Verification items for the finished model (mm, model axes). A direction names the side the tool comes from. Coordinates: 2 decimals unless noted, no trailing zeros. Write each loop counter-clockwise with the first axis right and the second up, starting at its lowest first coordinate (ties: lowest second). Pieces come first, ordered by that corner, then holes.
```python
from build123d import *

# Parameters (mm, degrees)
F1_DEPTH     = 10
F2_R         = 2
F3_DEPTH     = 115.001
F4_R         = 2
F4_R_2       = 1.25
F5_DEPTH     = 5
F6_R         = 2
F7_DEPTH     = 5
F9_DEPTH     = 10
F10_R        = 4.99999
F11_R        = 5
F12_DEPTH    = 10.001
F14_DEPTH    = 10
F15_T4_DEPTH = 78.4438958161
F15_T9_DEPTH = 78.4438958161
F16_R        = 4.99999


# Not quite as in the source:
# - a fillet or chamfer that OpenCascade refuses, or shapes differently, is made with other operations: its cross-section is extruded or revolved along the edge and cut away or added
# - a fillet or chamfer is up to 0.001 mm smaller than in the source, because OpenCascade refuses the exact size


with BuildPart() as f1:
    # F0 (on Front) → F1 (new body)
    with BuildSketch(Plane.XZ):
        Polygon((0, 115), (0, 0), (10, 0), (20, 0), (20, 5), (10, 5), (10, 110), (20, 110), (20, 115), (10, 115), align=None)
    extrude(amount=F1_DEPTH)

    # F2 (on face) → F3 (cut, through all)
    with BuildSketch(Plane.XY.offset(115)):
        with BuildLine():
            Line((0, -10), (5, -10))
            ThreePointArc((5, -10), (1.4644660941, -8.5355339059), (0, -5))
            Line((0, -5), (0, -10))
        make_face()
        with BuildLine():
            Line((0, 0), (0, -5))
            ThreePointArc((0, -5), (1.4644660941, -1.4644660941), (5, 0))
            Line((5, 0), (0, 0))
        make_face()
        with BuildLine():
            ThreePointArc((15.2, 0), (18.5941125497, -1.4058874503), (20, -4.8))
            Line((20, -4.8), (20, 0))
            Line((20, 0), (15.2, 0))
        make_face()
        with BuildLine():
            ThreePointArc((20, -5), (18.5355339059, -8.5355339059), (15, -10))
            Line((15, -10), (20, -10))
            Line((20, -10), (20, -5))
        make_face()
        with Locations((15, -5)):
            Circle(F2_R)
    extrude(amount=-F3_DEPTH, mode=Mode.SUBTRACT)

    # F4 (on face) → F5 (join)
    with BuildSketch(Plane.XY.offset(115)):
        with Locations((15, -5)):
            Circle(F4_R)
        with Locations((15, -5)):
            Circle(F4_R_2, mode=Mode.SUBTRACT)
    extrude(amount=-F5_DEPTH)

    # F6 (on face) → F7 (join)
    with BuildSketch(Plane(origin=(0, 0, 0), x_dir=(1, 0, 0), z_dir=(0, 0, -1))):
        with BuildLine():
            Line((-25, 0), (5, 0))
            ThreePointArc((5, 0), (0, 5), (5, 10))
            Line((5, 10), (-25, 10))
            ThreePointArc((-25, 10), (-28.5355339059, 8.5355339059), (-30, 5))
            ThreePointArc((-30, 5), (-28.5355339059, 1.4644660941), (-25, 0))
        make_face()
        with Locations((-25, 5)):
            Circle(F6_R, mode=Mode.SUBTRACT)
    extrude(amount=-F7_DEPTH)

    # F8 (on face) → F9 (join)
    with BuildSketch(Plane.XZ.offset(10)):
        Polygon((0, 115), (-20, 5), (5, 5), (5, 115), align=None)
    extrude(amount=-F9_DEPTH)

    # F10 (radius 5 in the source; OpenCascade refuses exactly that, so slightly less here)
    f10_edges = [f1.edges().sort_by_distance(p)[0] for p in [
        (-10, 0, 60),
        (-10, -10, 60),
    ]]
    fillet(f10_edges, radius=F10_R)

    # F11 (on face) → F12 (cut, through all)
    with BuildSketch(Plane.XZ.offset(10)):
        with Locations((0, 50.3422953188)):
            Circle(F11_R)
    extrude(amount=-F12_DEPTH, mode=Mode.SUBTRACT)

    # F13 (on face) → F14 (join)
    with BuildSketch(Plane(origin=(0, 0, 0), x_dir=(-1, 0, 0), z_dir=(0, 1, 0))):
        Polygon((-20, 110), (-10, 57.5), (-10, 110), (-15.2, 110), align=None)
    extrude(amount=-F14_DEPTH)

    # F15: fillet of radius 5 on 2 edges, made by hand


with BuildPart() as f15_tool2:
    # F15_s3 → F15_t4 (new body)
    with BuildSketch(Plane(origin=(23.2579385477, 0, 122.1041773757), x_dir=(0, 1, 0), z_dir=(-0.1871121079, 0, -0.9823385664))):
        with BuildLine():
            ThreePointArc((0, -5.9355605394), (-1.4644660941, -2.4000266335), (-5, -0.9355605394))
            Line((-5, -0.9355605394), (0, -0.9355605394))
            Line((0, -0.9355605394), (0, -5.9355605394))
        make_face()
    extrude(amount=F15_T4_DEPTH)

    split(bisect_by=Plane.YZ.offset(10), keep=Keep.TOP)


with BuildPart() as f1_1:
    add(f1.part)

    # F15_t1: cut F15_tool2
    add(f15_tool2.part, mode=Mode.SUBTRACT)


with BuildPart() as f15_tool7:
    # F15_s8 → F15_t9 (new body)
    with BuildSketch(Plane(origin=(23.2579385477, 0, 122.1041773757), x_dir=(0, 1, 0), z_dir=(-0.1871121079, 0, -0.9823385664))):
        with BuildLine():
            ThreePointArc((-10, -5.9355605394), (-8.5355339059, -2.4000266335), (-5, -0.9355605394))
            Line((-5, -0.9355605394), (-10, -0.9355605394))
            Line((-10, -0.9355605394), (-10, -5.9355605394))
        make_face()
    extrude(amount=F15_T9_DEPTH)

    split(bisect_by=Plane.YZ.offset(10), keep=Keep.TOP)


with BuildPart() as f1_2:
    add(f1_1.part)

    # F15_t6: cut F15_tool7
    add(f15_tool7.part, mode=Mode.SUBTRACT)

    # F16 (radius 5 in the source; OpenCascade refuses exactly that, so slightly less here)
    f16_edges = [f1_2.edges().sort_by_distance(p)[0] for p in [
        (10, 0, 44.610974),
        (10, -10, 44.610974),
    ]]
    fillet(f16_edges, radius=F16_R)


solid = f1_2.part
```
1. Material ranges on L1, parallel to Y at x = 15, z = 113; L2, parallel to Y at x = 15, z = 2; L3, parallel to X at y = -8.5, z = 53, recorded low to high.
2. Tool access check on faces 4 (the cylindrical face through (9, -8, 31)), 5 (the flat face through (15, -5, 110)), 6 (the cylindrical face through (-1.08, -5.07, 45.46)). Record the directions out of +Z, -Z, +X, -X, +Y, -Y that give a thin tool (end or side, any length) a straight path to the whole face; none if there is none.
3. Gauge pin test, flat ends, axial feed: P1, Ø5, axis at x = -25, y = -5, coming from the +Z side; P2, Ø4, axis at y = -8, z = 35.5, coming from the -X side; P3, Ø3, axis at y = -2.5, z = 35.5, coming from the -X side. Record the tip position at first contact, or that the pin passes through.
4. Sectioned sample at A-A, the plane y = -8.5. Record the boundary of the cut face in (x, z).
5. Draft check along X on faces 1 (the flat face through (10, -5, 115)), 2 (the cylindrical face through (9, -2, 32)), 3 (the cylindrical face through (13.4, -6.2, 2.5)). Enter one of: pulls with the +X half, pulls with the -X half, needs draft (parallel to the pull), parting line crosses it, or undercut.
Outcome:
1. L1: y = -10 to -6.25, -3.75 to 0
1. L2: y = -10 to -7, -3 to 0
1. L3: x = -9.82 to -4.24, 4.24 to 8.57
2. face 4: +X, -Y
2. face 5: +Z
2. face 6: +Y, -Y
3. P1: stops at z = 5
3. P2: stops at x = -14.47
3. P3: stops at x = -14.44
4. outline: (-28.57, 0) - (18.57, 0) - (18.57, 5) - (8.57, 5) - (8.57, 57.63) - (18.57, 110.13) - (18.57, 115) - (1.45, 115) - (-18.55, 5) - (-28.57, 5) - close; hole circle Ø10 at (0, 50.34)
5. face 1: needs draft
5. face 2: pulls with the +X half
5. face 3: undercut
